```python
from build123d import *

# Parameters (mm, degrees)
MM_1_D              = 6
MM_1_DEPTH          = 4
MM_1_TIP            = 1.802581857
CUT_EXTRUDE_1_DEPTH = 4
FILLET_1_R          = 0.2
CHAMFER_1_SIZE      = 0.6
FILLET_2_R          = 0.4


with BuildPart() as part:
    # 草图1 → 旋转1 (revolve)
    with BuildSketch(Plane.XY):
        Polygon((0, 0), (0, 6.5), (8, 6.5), (8, 4), (23, 4), (23, 0), align=None)
    revolve(axis=Axis((0, 0, 0), (1, 0, 0)))

    # 大小mm 暗销孔1
    with Locations(Plane.ZY):
        with Locations((0, 0)):
            Hole(MM_1_D / 2, depth=MM_1_DEPTH)
            with Locations((0, 0, -(MM_1_DEPTH + MM_1_TIP / 2))):  # 118° drill point
                Cone(0, MM_1_D / 2, MM_1_TIP, mode=Mode.SUBTRACT)

    # 草图4 → 切除-拉伸1 (cut)
    with BuildSketch(Plane.ZY):
        Polygon((3, 1.732050808), (0, 3.464101615), (-3, 1.732050808), (-3, -1.732050808), (0, -3.464101615), (3, -1.732050808), align=None)
    extrude(amount=-CUT_EXTRUDE_1_DEPTH, mode=Mode.SUBTRACT)

    # 圆角1
    fillet_1_edges = [part.edges().sort_by_distance(p)[0] for p in [
        (0, -6.5, 0),
    ]]
    fillet(fillet_1_edges, radius=FILLET_1_R)

    # 倒角1
    chamfer_1_edges = [part.edges().sort_by_distance(p)[0] for p in [
        (23, -4, 0),
    ]]
    chamfer(chamfer_1_edges, length=CHAMFER_1_SIZE)

    # 圆角2
    fillet_2_edges = [part.edges().sort_by_distance(p)[0] for p in [
        (8, -4, 0),
    ]]
    fillet(fillet_2_edges, radius=FILLET_2_R)


solid = part.part
```
Can you work these out from the model? Positions are in its coordinate system, mm. A direction names the side the tool comes from. Round coordinates to 2 decimals unless told otherwise and drop trailing zeros. Loops run counter-clockwise (first coordinate to the right, second up) from the corner with the lowest first, then second, coordinate; pieces in that order, holes last. Notation, with made-up numbers: (-14, 67.25) -> (17, 67.25) arc R26 cw to (17, 101.25) -> close; hole circle Ø3 at (-11.5, -18.75). An arc over 180 degrees is marked (long way). One line per item, written item: value. Start each with the question number.
1. If I drill on probe 1 along X at (y, z) = (4.75, 2.5); probe 2 along Z at (x, y) = (7.75, -0.25); probe 3 along Z at (x, y) = (3, -2.25), over which ranges is the centre line in solid material (lowest first)?
2. For faces 5 (the flat face through (2, 0, -3)), 6 (the flat face through (23, 0, 0)), which set-ups out of +Z, -Z, +X, -X, +Y, -Y let a thin tool reach every point of the face, with its end or its side?
3. For pin 1 (1.2 mm diameter, centred on y = -2, z = 2, fed in from -X); pin 2 (1.5 mm diameter, centred on x = 2.5, y = -5, fed in from +Z); pin 3 (6 mm diameter, centred on x = 19, z = 0, fed in from +Y); pin 4 (4 mm diameter, centred on x = 7, y = 3.5, fed in from +Z), each with a flat end and sliding along its axis, tell me the tip position at first contact or that it passes through.
4. If we section it at A-A, the plane x = 6.5: Write out the boundary of the cut face in (y, z).
5. If we mould it in two halves opening along Y, with no side actions, what happens to faces 1 (the flat face through (0, 2.9, -1.3)), 2 (the flat face through (2, -2.6, 1.5)), 3 (the cylindrical face through (15.498, -0.867, -3.905)), 4 (the flat face through (4, 1.5, -2.8))? For each: pulls with the +Y half, pulls with the -Y half, needs draft (parallel to the pull), parting line crosses it, or undercut.
6. If we section it at B-B, the plane x = 17.25: Write out the boundary of the cut face in (y, z).
Calculated:
1. probe 1: x = 0 to 8
1. probe 2: z = -6.5 to 6.5
1. probe 3: z = -6.1 to -2.1, 2.1 to 6.1
2. face 5: -X
2. face 6: +Z, -Z, +X, +Y, -Y
3. pin 1: stops at x = 0
3. pin 2: stops at z = 4.92
3. pin 3: stops at y = 4
3. pin 4: stops at z = 6.32
4. outline: circle Ø13 at (0, 0)
5. face 1: needs draft
5. face 2: undercut
5. face 3: parting line crosses it
5. face 4: undercut
6. outline: circle Ø8 at (0, 0)
